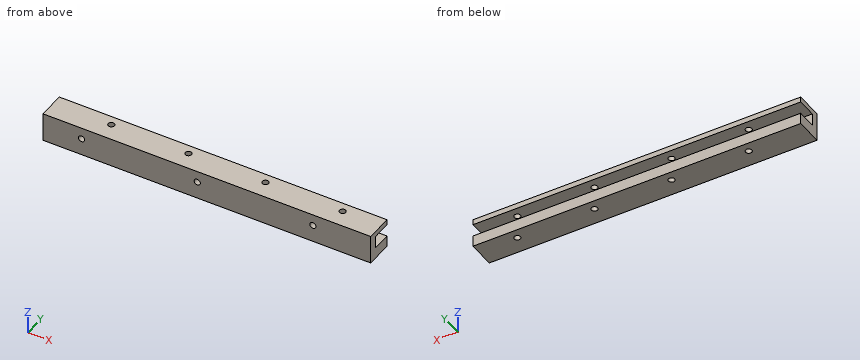
Autodesk Inventor part; units mm, degrees
ref_plane "YZ Plane" through (0, 0, 0) normal (1, 0, 0) x (0, 1, 0)
ref_plane "XZ Plane" through (0, 0, 0) normal (0, 1, 0) x (-1, 0, 0)
ref_plane "XY Plane" through (0, 0, 0) normal (0, 0, 1) x (1, 0, 0)
sketch "スケッチ1" plane through (0, 0, 0) normal (0, 1, 0) x (-1, 0, 0)
  line L0 (-90, -3) -> (90, -3)
  line L1 (90, -3) -> (90, 3)
  line L2 (90, 3) -> (-90, 3)
  line L3 (-90, 3) -> (-90, -3)
  line L4 (-90, -3) -> (90, 3) construction
  line L5 (90, -3) -> (-90, 3) construction
  point P0 (0, 0)
  dimension "d0" = 180
  dimension "d1" = 6
extrude "押し出し1" add sketch "スケッチ1" along normal blind 17
sketch "スケッチ2" plane through (0, 0, 0) normal (0, -1, 0) x (1, 0, 0)
  line L0 (-90, 3) -> (90, 3)
  line L1 (90, 3) -> (-80, 3)
  line L2 (-80, 3) -> (-80, 9)
  line L3 (-80, 9) -> (90, 9)
  line L4 (90, 9) -> (90, 3)
  line L5 (90, 3) -> (90, -3)
  line L6 (90, -3) -> (-80, -3)
  line L7 (-80, -3) -> (-80, -6)
  line L8 (-80, -6) -> (90, -6)
  line L9 (90, -6) -> (90, -3)
  point P0 (0, 0)
  dimension "d4" = 170
  dimension "d5" = 6
  dimension "d6" = 170
  dimension "d7" = 3
extrude "押し出し2" add sketch "スケッチ2" against normal blind 14
sketch "スケッチ3" plane through (0, 17, 0) normal (0, 1, 0) x (1, 0, 0)
  line L0 (-90, 3) -> (-90, -3)
  line L1 (90, -3) -> (90, 3)
  line L2 (-90, 3) -> (90, 3)
  line L3 (90, 3) -> (90, -3)
  line L4 (90, -3) -> (-90, -3)
  line L5 (-90, -3) -> (-90, 3)
  point P0 (0, 0)
extrude "押し出し3" cut sketch "スケッチ3" against normal blind 13
sketch "スケッチ4" plane through (0, 4, 0) normal (0, 1, 0) x (1, 0, 0)
  line L0 (-90, -3) -> (-90, 3)
  line L1 (-80, 6) -> (-80, 3)
  line L2 (-90, -3) -> (-80, -3)
  line L3 (-80, -3) -> (-80, 3)
  line L4 (-80, 3) -> (-90, 3)
  line L5 (-90, 3) -> (-90, -3)
  point P0 (0, 0)
extrude "押し出し4" cut sketch "スケッチ4" against normal blind 13
sketch "スケッチ5" plane through (0, 14, 0) normal (0, 1, 0) x (1, 0, 0)
  line L0 (97.0492, -3.2) -> (-97.0492, -3.2)
  line L1 (-97.0492, -3.2) -> (-97.0492, 3.2)
  line L2 (-97.0492, 3.2) -> (97.0492, 3.2)
  line L3 (97.0492, 3.2) -> (97.0492, -3.2)
  line L4 (97.0492, -3.2) -> (-97.0492, 3.2) construction
  line L5 (-97.0492, -3.2) -> (97.0492, 3.2) construction
  point P0 (0, 0)
  dimension "d14" = 6.4
extrude "押し出し5" cut sketch "スケッチ5" against normal blind 10
sketch "スケッチ6" plane through (-80, 0, 9) normal (0, 0, 1) x (1, 0, 0)
  line L0 (0, 14) -> (170, 14)
  line L1 (170, 0) -> (170, 14)
  point P0 (80, 0)
  point P1 (150, 9)
  point P2 (110, 9)
  point P3 (70, 9)
  point P4 (30, 9)
  dimension "d17" = 5
  dimension "d18" = 20
  dimension "d19" = 40
  dimension "d20" = 5
  dimension "d21" = 40
  dimension "d22" = 40
hole "穴1" at (70, 9, 9) at (30, 9, 9) at (-10, 9, 9) at (-50, 9, 9) direction (0, 0, -1) diameter 3.2 end through all
sketch "スケッチ7" plane through (0, 0, 0) normal (0, -1, 0) x (1, 0, 0)
  line L0 (-80, -6) -> (90, -6)
  line L1 (90, -6) -> (90, 9)
  line L2 (-80, -3.2) -> (90, -3.2)
  point P0 (0, 0)
  point P1 (60, 0)
  point P2 (0, 0)
  point P3 (-60, 0)
  dimension "d30" = 6
  dimension "d31" = 30
  dimension "d32" = 60
hole "穴2" at (60, 0, 0) at (0, 0, 0) at (-60, 0, 0) direction (0, 1, 0) diameter 3.2 end through all
sketch "スケッチ8" plane through (90, 0, -6) normal (0, 0, -1) x (-1, 0, 0)
  line L0 (170, 0) -> (170, 14)
  line L1 (0, 0) -> (170, 0)
  line L2 (170, 0) -> (170, 14)
  line L3 (170, 14) -> (0, 14)
  line L4 (0, 14) -> (0, 0)
  point P0 (90, 0)
extrude "押し出し6" add sketch "スケッチ8" along normal blind 3
sketch "スケッチ10" plane through (-80, 0, 9) normal (0, 0, 1) x (1, 0, 0)
  circle A0 centre (150, 9) radius 1.6
  circle A1 centre (110, 9) radius 1.6
  circle A2 centre (70, 9) radius 1.6
  circle A3 centre (30, 9) radius 1.6
  point P0 (80, 0)
hole "穴3" at (70, 9, 9) at (30, 9, 9) at (-10, 9, 9) at (-50, 9, 9) direction (0, 0, -1) diameter 3.2 end through all
sketch "スケッチ11" plane through (0, 14, 0) normal (0, 1, 0) x (1, 0, 0)
  line L0 (-80, -9) -> (90, -9)
  line L1 (-80, -9) -> (90, -9)
  line L2 (90, -9) -> (90, -6)
  line L3 (90, -6) -> (-80, -6)
  line L4 (-80, -6) -> (-80, -9)
  point P0 (0, 0)
  dimension "d49" = 170
  dimension "d50" = 3
extrude "押し出し7" cut sketch "スケッチ11" against normal blind 40
properties part number "lock2"
The listing builds one solid part. Answer for the finished solid, in the listing's coordinates (mm). Give positions to 0.01 mm unless a question says otherwise; leave off trailing zeros. Loops run counter-clockwise (first coordinate to the right, second up) from the corner with the lowest first, then second, coordinate; pieces in that order, holes last. Notation, with made-up numbers: M 29,-16.75 L 84,-16.75 A18 cw 84,-11.75 Z; hole C 28.5,37 d7. An arc over 180 degrees is marked long. One line per item, written item: value.
1. Section C-C on z = 0 is taken. Determine the outline of the cut face in (x, y), plus the area to 3 significant figures.
Found:
outline: M -80,0 L -61.6,0 L -61.6,4 L -80,4 Z; M -58.4,0 L -1.6,0 L -1.6,4 L -58.4,4 Z; M 1.6,0 L 58.4,0 L 58.4,4 L 1.6,4 Z; M 61.6,0 L 90,0 L 90,4 L 61.6,4 Z
area: 642 mm^2
2. Find the intervals of material crossed by probe 1 along X at (y, z) = (9, 4.4); probe 2 along X at (y, z) = (1.5, 0); probe 3 along Z at (x, y) = (6, 11.25), in increasing order.
Found:
probe 1: -80 to -51.6, -48.4 to -11.6, -8.4 to 28.4, 31.6 to 68.4, 71.6 to 90
probe 2: -80 to -61.6, -58.4 to -1.6, 1.6 to 58.4, 61.6 to 90
probe 3: -9 to -3.2, 3.2 to 6
3. Each of these flat-tipped pins is pushed along its axis until it touches: P1, Ø1.5, axis at y = 12.5, z = -1.5, coming from the +X side; P2, Ø1.9, axis at x = -26.5, z = -0.5, coming from the +Y side. Where does it stop, or does it pass through?
Found:
P1: through
P2: y = 4
4. Section A-A on x = -50 is taken. Determine the outline of the cut face in (y, z), plus the area to 3 significant figures.
Found:
outline: M 0,-9 L 7.4,-9 L 7.4,-3.2 L 4,-3.2 L 4,3.2 L 7.4,3.2 L 7.4,6 L 0,6 Z; M 10.6,-9 L 14,-9 L 14,-3.2 L 10.6,-3.2 Z; M 10.6,3.2 L 14,3.2 L 14,6 L 10.6,6 Z
area: 118 mm^2
5. Section B-B on y = 5.5 is taken. Determine the outline of the cut face in (x, z).
Found:
outline: M -80,-9 L 90,-9 L 90,-3.2 L -80,-3.2 Z; M -80,3.2 L 90,3.2 L 90,6 L -80,6 Z
6. Section D-D on x = 25 is taken. Determine the outline of the cut face in (y, z).
Found:
outline: M 0,-9 L 14,-9 L 14,-3.2 L 4,-3.2 L 4,3.2 L 14,3.2 L 14,6 L 0,6 Z
